from build123d import *

# Parameters (mm, degrees)
SKETCH_W     = 48.25
SKETCH_H     = 81.5
SKETCH_R     = 2.65
PAD_DEPTH    = 8
POCKET_DEPTH = 4
FILLET_R     = 4


with BuildPart() as part:
    # Sketch → Pad (new body)
    with BuildSketch(Plane.XY):
        Rectangle(SKETCH_W, SKETCH_H)
        with Locations((13.335, 28.32)):
            Circle(SKETCH_R, mode=Mode.SUBTRACT)
        with Locations((-13.335, -28.32)):
            Circle(SKETCH_R, mode=Mode.SUBTRACT)
    extrude(amount=PAD_DEPTH)

    # Sketch001 (on Face8 of Pad) → Pocket (cut)
    with BuildSketch(Plane.XY.offset(8)):
        Polygon((17.285, 26.039466), (17.285, 30.600534), (13.335, 32.881067), (9.385, 30.600534), (9.385, 26.039466), (13.335, 23.758933), align=None)
        Polygon((-9.385, -26.039466), (-13.335, -23.758933), (-17.285, -26.039466), (-17.285, -30.600534), (-13.335, -32.881067), (-9.385, -30.600534), align=None)
    extrude(amount=-POCKET_DEPTH, mode=Mode.SUBTRACT)

    # Fillet
    fillet_edges = [part.edges().sort_by_distance(p)[0] for p in [
        (-24.125, -40.75, 4),
        (24.125, -40.75, 4),
        (24.125, 40.75, 4),
        (-24.125, 40.75, 4),
    ]]
    fillet(fillet_edges, radius=FILLET_R)


solid = part.part
Read the model definition and answer for the solid it produces. Units are mm, in the model's axes. A direction names the side the tool comes from. Coordinates: 2 decimals unless noted, no trailing zeros. Write each loop counter-clockwise with the first axis right and the second up, starting at its lowest first coordinate (ties: lowest second). Pieces come first, ordered by that corner, then holes. Notation, with made-up numbers: M 52.25,79 L 78.25,79 A30 ccw 78.25,103 Z; hole C 64.5,18.25 d7. An arc over 180 degrees is marked long. Use a Markdown table: item, result.
Q1. The part is cut by section B-B, the plane z = 5. Write down the section's boundary in (x, y) (3 decimals).
Answer block:
| item | result |
|---|---|
| outline | M -24.125,-36.75 A4 ccw -20.125,-40.75 L 20.125,-40.75 A4 ccw 24.125,-36.75 L 24.125,36.75 A4 ccw 20.125,40.75 L -20.125,40.75 A4 ccw -24.125,36.75 Z; hole M -17.285,-30.601 L -13.335,-32.881 L -9.385,-30.601 L -9.385,-26.039 L -13.335,-23.759 L -17.285,-26.039 Z; hole M 9.385,26.039 L 13.335,23.759 L 17.285,26.039 L 17.285,30.601 L 13.335,32.881 L 9.385,30.601 Z |
Q2. Determine the mould class of faces 3 (the face through (-15.338, -31.725, 6.028)), 4 (the face through (-16, -29.3, 4)), 5 (the face through (0, 40.75, 4)), 6 (the face through (0, 1, 0)) for opening direction Y: released by +Y, released by -Y, zero draft, split by the parting line, or undercut.
Answer block:
| item | result |
|---|---|
| face 3 | undercut |
| face 4 | undercut |
| face 5 | released by +Y |
| face 6 | zero draft |
Q3. Which of the six approach directions +Z, -Z, +X, -X, +Y, -Y give full straight-line access (tool end or side, diameter ignored) to faces 1 (the face through (-15.28, -24.88, 6.03)), 2 (the face through (22.92, -39.61, 4.06))?
Answer block:
| item | result |
|---|---|
| face 1 | +Z |
| face 2 | +Z, -Z, +X, -Y |
Q4. Straight lines are drawn through the part: L1, parallel to X at y = -28.5, z = 6 (3 decimals); L2, parallel to X at y = -28.32, z = 1.95 (3 decimals); L3, parallel to Y at x = -15.5, z = 6.5. For each, find the intervals that lie inside material, in ascending order. Write a range as [from, to].
Answer block:
| item | result |
|---|---|
| L1 | x = [-24.125, -17.285], [-9.385, 24.125] |
| L2 | x = [-24.125, -15.985], [-10.685, 24.125] |
| L3 | y = [-40.75, -31.63], [-25.01, 40.75] |
Q5. This flat-tipped pin is pushed along its axis until it touches: pin 1 Ø7 at (x, y) = (13.335, 28.32) entering from +Z. Where does it stop, or does it pass through?
Answer block:
| item | result |
|---|---|
| pin 1 | stops at z = 4 |
Q6. The part is cut by section A-A, the plane y = 28.32. Write down the section's boundary in (x, z) (3 decimals).
Answer block:
| item | result |
|---|---|
| outline | M -24.125,0 L 10.685,0 L 10.685,4 L 9.385,4 L 9.385,8 L -24.125,8 Z; M 15.985,0 L 24.125,0 L 24.125,8 L 17.285,8 L 17.285,4 L 15.985,4 Z |
Q7. The part is cut by section C-C, the plane x = 12. Write down the section's boundary in (y, z).
Answer block:
| item | result |
|---|---|
| outline | M -40.75,0 L 26.03,0 L 26.03,4 L 24.53,4 L 24.53,8 L -40.75,8 Z; M 30.61,0 L 40.75,0 L 40.75,8 L 32.11,8 L 32.11,4 L 30.61,4 Z |
